CAD build for the part. Positions are in the model's coordinates, mm. Face numbers are marked on the shaded views. A direction names the side the tool comes from. Give positions to 0.01 mm unless a question says otherwise; leave off trailing zeros. Write each loop counter-clockwise with the first axis right and the second up, starting at its lowest first coordinate (ties: lowest second). Pieces come first, ordered by that corner, then holes. Notation, with made-up numbers: (64, -2) - (100, -2) arc R12 ccw to (100, 19) - close; hole circle Ø7 at (7.5, 49.5). An arc over 180 degrees is marked (long way). Put each result on its own line as item: value. Start each with the question number.
1. Cut at C-C on z = 56.5. List the corners of the cut face in (x, y), and give its area (3 significant figures).
2. Cut at A-A on x = 40. List the corners of the cut face in (y, z).
3. Tool access for the marked faces 1, 2 and 3: list every direction of +Z, -Z, +X, -X, +Y, -Y with a clear straight run to the whole face (end or side of a thin tool).
4. Cut at D-D on x = 53.5. List the corners of the cut face in (y, z).
5. Drop flat-ended pins along their axis: pin 1 (8 mm diameter, centred on y = 66, z = 23, fed in from +X); pin 2 (1.5 mm diameter, centred on x = 36, z = 25.5, fed in from -Y); pin 3 (10 mm diameter, centred on y = 39, z = 60, fed in from -X). Give the stop position or say it passes through.
6. Wall check: line 1 (Z direction, x = 5, y = 16); line 2 (Y direction, x = 32.5, z = 49); line 3 (Y direction, x = 52, z = 13). Give the ranges that are in metal, low to high.
7. Cut at B-B on y = 69.5. List the corners of the cut face in (x, z).
Autodesk Inventor part; units mm, degrees
ref_plane "YZ Plane" through (0, 0, 0) normal (1, 0, 0) x (0, 1, 0)
ref_plane "XZ Plane" through (0, 0, 0) normal (0, 1, 0) x (-1, 0, 0)
ref_plane "XY Plane" through (0, 0, 0) normal (0, 0, 1) x (1, 0, 0)
sketch "Sketch1" plane through (0, 0, 0) normal (0, 0, 1) x (1, 0, 0)
  line L0 (0, 0) -> (80, 0)
  line L1 (80, 0) -> (80, 80)
  line L2 (80, 80) -> (0, 80)
  line L3 (0, 80) -> (0, 0)
  dimension "d0" = 80
  dimension "d1" = 80
extrude "Extrusion1" add sketch "Sketch1" along normal blind 6
sketch "Sketch2" plane through (0, 0, 6) normal (0, 0, 1) x (1, 0, 0)
  line L0 (80, 80) -> (0, 80)
  line L1 (0, 80) -> (0, 0)
  arc A0 (65, 40) -> (15, 40) centre (40, 40) ccw
  line L2 (15, 40) -> (65, 40)
  dimension "d4" = 50
  dimension "d5" = 40
  dimension "d6" = 40
extrude "Extrusion2" add sketch "Sketch2" along normal blind 80
properties part number "SpoolHolder"
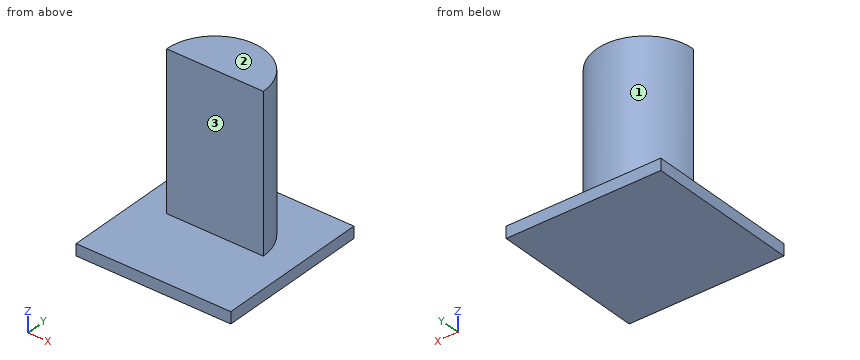
Report:
1. outline: (15, 40) - (65, 40) arc R25 ccw to start
1. area: 982 mm²
2. outline: (0, 0) - (80, 0) - (80, 6) - (65, 6) - (65, 86) - (40, 86) - (40, 6) - (0, 6) - close
3. face 1: +Z, +Y
3. face 2: +Z, +X, -X, +Y, -Y
3. face 3: +Z, +X, -X, -Y
4. outline: (0, 0) - (80, 0) - (80, 6) - (61.04, 6) - (61.04, 86) - (40, 86) - (40, 6) - (0, 6) - close
5. pin 1: stops at x = 51.87
5. pin 2: stops at y = 40
5. pin 3: stops at x = 15
6. line 1: z = 0 to 6
6. line 2: y = 40 to 63.85
6. line 3: y = 40 to 61.93
7. outline: (0, 0) - (80, 0) - (80, 6) - (0, 6) - close
